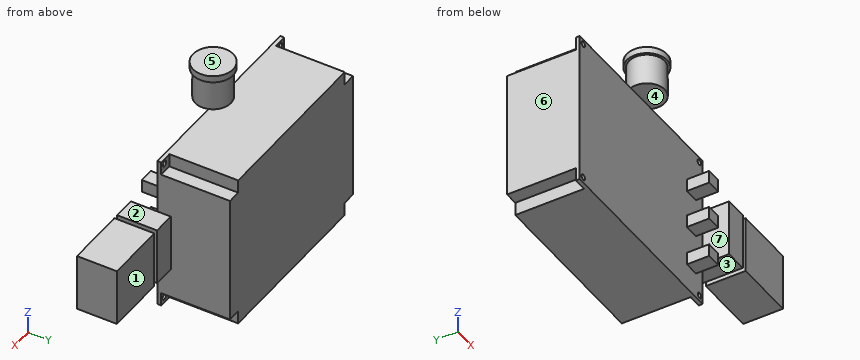
```python
from build123d import *

# Parameters (mm, degrees)
SKETCH2_W               = 90
SKETCH2_H               = 70
BOSS_EXTRUDE1_DEPTH     = 32.6
SKETCH4_R               = 8
BOSS_EXTRUDE2_DEPTH     = 14
SKETCH6_W               = 6.6
SKETCH6_H               = 5.7
BOSS_EXTRUDE3_DEPTH     = 10
SKETCH10_W              = 6.6
SKETCH10_H              = 5.7
BOSS_EXTRUDE4_DEPTH     = 10
SKETCH7_W               = 6.6
SKETCH7_H               = 5.7
BOSS_EXTRUDE5_DEPTH     = 10
CUT_EXTRUDE1_DEPTH      = 122.916565322
CUT_EXTRUDE1_DEPTH_BACK = 122.916565322
SKETCH11_R              = 1.25
CUT_EXTRUDE2_DEPTH      = 122.916565322
CUT_EXTRUDE2_DEPTH_BACK = 122.916565322
SKETCH15_R              = 1.25
CUT_EXTRUDE3_DEPTH      = 122.916565322
CUT_EXTRUDE3_DEPTH_BACK = 122.916565322
SKETCH14_R              = 1.25
CUT_EXTRUDE4_DEPTH      = 122.916565322
CUT_EXTRUDE4_DEPTH_BACK = 122.916565322
SKETCH12_R              = 1.25
SKETCH16_W              = 6
SKETCH16_H              = 6
CUT_EXTRUDE5_DEPTH      = 30.9
SKETCH19_W              = 6
SKETCH19_H              = 6
CUT_EXTRUDE6_DEPTH      = 30.9
SKETCH18_W              = 6
SKETCH18_H              = 6
CUT_EXTRUDE7_DEPTH      = 30.9
SKETCH17_W              = 6
SKETCH17_H              = 6
CUT_EXTRUDE8_DEPTH      = 30.9
SKETCH20_W              = 25.8
SKETCH20_H              = 17.9
BOSS_EXTRUDE6_DEPTH     = 39.4
SKETCH22_W              = 2.1
SKETCH22_H              = 17.9
CUT_EXTRUDE9_DEPTH      = 2.75
SKETCH24_W              = 2.1
SKETCH24_H              = 25.8
CUT_EXTRUDE10_DEPTH     = 2.75
SKETCH25_W              = 2.1
SKETCH25_H              = 17.9
CUT_EXTRUDE11_DEPTH     = 2.75
SKETCH26_W              = 2.1
SKETCH26_H              = 25.8
CUT_EXTRUDE12_DEPTH     = 2.75
SKETCH27_R              = 9
BOSS_EXTRUDE7_DEPTH     = 3


with BuildPart() as part:
    # Sketch2 → Boss-Extrude1 (new body)
    with BuildSketch(Plane(origin=(0, 0, 0), x_dir=(1, 0, 0), z_dir=(0, 1, 0))):
        with Locations((45, 35)):
            Rectangle(SKETCH2_W, SKETCH2_H)
    extrude(amount=BOSS_EXTRUDE1_DEPTH)

    # Sketch4 → Boss-Extrude2 (add)
    with BuildSketch(Plane.XY):
        with Locations(Location((45, -2.57, 0), (0, 0, 161.261463564))):
            Circle(SKETCH4_R)
    extrude(amount=BOSS_EXTRUDE2_DEPTH)

    # Sketch6 → Boss-Extrude3 (add)
    with BuildSketch(Plane(origin=(0, 0, 0), x_dir=(-1, 0, 0), z_dir=(0, -1, 0))):
        with Locations((-81.82, 55.55)):
            Rectangle(SKETCH6_W, SKETCH6_H)
    extrude(amount=BOSS_EXTRUDE3_DEPTH)

    # Sketch10 → Boss-Extrude4 (add)
    with BuildSketch(Plane.XZ):
        with Locations((81.82, -37.25)):
            Rectangle(SKETCH10_W, SKETCH10_H)
    extrude(amount=BOSS_EXTRUDE4_DEPTH)

    # Sketch7 → Boss-Extrude5 (add)
    with BuildSketch(Plane.XZ):
        with Locations((81.82, -19.65)):
            Rectangle(SKETCH7_W, SKETCH7_H)
    extrude(amount=BOSS_EXTRUDE5_DEPTH)

    # Sketch11 → Cut-Extrude1 (cut, two sides: drawn at the far end of the back side and taken through both)
    with BuildSketch(Plane(origin=(0, 32.6, 0), x_dir=(1, 0, 0), z_dir=(0, 1, 0)).offset(-CUT_EXTRUDE1_DEPTH_BACK)):
        with Locations(Location((87.55, 2.29, 0), (0, 0, 90))):
            Circle(SKETCH11_R)
    extrude(amount=CUT_EXTRUDE1_DEPTH + CUT_EXTRUDE1_DEPTH_BACK, mode=Mode.SUBTRACT)

    # Sketch15 → Cut-Extrude2 (cut, two sides: drawn at the far end of the back side and taken through both)
    with BuildSketch(Plane(origin=(0, 32.6, 0), x_dir=(1, 0, 0), z_dir=(0, 1, 0)).offset(-CUT_EXTRUDE2_DEPTH_BACK)):
        with Locations(Location((2.61, 67.35, 0), (0, 0, 90))):
            Circle(SKETCH15_R)
    extrude(amount=CUT_EXTRUDE2_DEPTH + CUT_EXTRUDE2_DEPTH_BACK, mode=Mode.SUBTRACT)

    # Sketch14 → Cut-Extrude3 (cut, two sides: drawn at the far end of the back side and taken through both)
    with BuildSketch(Plane(origin=(0, 32.6, 0), x_dir=(1, 0, 0), z_dir=(0, 1, 0)).offset(-CUT_EXTRUDE3_DEPTH_BACK)):
        with Locations(Location((2.63, 2.25, 0), (0, 0, 90))):
            Circle(SKETCH14_R)
    extrude(amount=CUT_EXTRUDE3_DEPTH + CUT_EXTRUDE3_DEPTH_BACK, mode=Mode.SUBTRACT)

    # Sketch12 → Cut-Extrude4 (cut, two sides: drawn at the far end of the back side and taken through both)
    with BuildSketch(Plane(origin=(0, 32.6, 0), x_dir=(1, 0, 0), z_dir=(0, 1, 0)).offset(-CUT_EXTRUDE4_DEPTH_BACK)):
        with Locations(Location((87.71, 67.37, 0), (0, 0, 90))):
            Circle(SKETCH12_R)
    extrude(amount=CUT_EXTRUDE4_DEPTH + CUT_EXTRUDE4_DEPTH_BACK, mode=Mode.SUBTRACT)

    # Sketch16 → Cut-Extrude5 (cut)
    with BuildSketch(Plane(origin=(0, 32.6, 0), x_dir=(1, 0, 0), z_dir=(0, 1, 0))):
        with Locations((3, 67)):
            Rectangle(SKETCH16_W, SKETCH16_H)
    extrude(amount=-CUT_EXTRUDE5_DEPTH, mode=Mode.SUBTRACT)

    # Sketch19 → Cut-Extrude6 (cut)
    with BuildSketch(Plane(origin=(0, 32.6, 0), x_dir=(1, 0, 0), z_dir=(0, 1, 0))):
        with Locations((3, 3)):
            Rectangle(SKETCH19_W, SKETCH19_H)
    extrude(amount=-CUT_EXTRUDE6_DEPTH, mode=Mode.SUBTRACT)

    # Sketch18 → Cut-Extrude7 (cut)
    with BuildSketch(Plane(origin=(0, 32.6, 0), x_dir=(1, 0, 0), z_dir=(0, 1, 0))):
        with Locations((87, 3)):
            Rectangle(SKETCH18_W, SKETCH18_H)
    extrude(amount=-CUT_EXTRUDE7_DEPTH, mode=Mode.SUBTRACT)

    # Sketch17 → Cut-Extrude8 (cut)
    with BuildSketch(Plane(origin=(0, 32.6, 0), x_dir=(1, 0, 0), z_dir=(0, 1, 0))):
        with Locations((87, 67)):
            Rectangle(SKETCH17_W, SKETCH17_H)
    extrude(amount=-CUT_EXTRUDE8_DEPTH, mode=Mode.SUBTRACT)

    # Sketch20 → Boss-Extrude6 (add)
    with BuildSketch(Plane(origin=(90, 0, 0), x_dir=(0, 0, -1), z_dir=(1, 0, 0))):
        with Locations((37.6, -2.95)):
            Rectangle(SKETCH20_W, SKETCH20_H)
    extrude(amount=BOSS_EXTRUDE6_DEPTH)

    # Sketch22 → Cut-Extrude9 (cut)
    with BuildSketch(Plane(origin=(0, 0, -50.5), x_dir=(-1, 0, 0), z_dir=(0, 0, -1))):
        with Locations((-101.05, -2.95)):
            Rectangle(SKETCH22_W, SKETCH22_H)
    extrude(amount=-CUT_EXTRUDE9_DEPTH, mode=Mode.SUBTRACT)

    # Sketch24 → Cut-Extrude10 (cut)
    with BuildSketch(Plane(origin=(0, 6, 0), x_dir=(1, 0, 0), z_dir=(0, 1, 0))):
        with Locations((101.05, 37.6)):
            Rectangle(SKETCH24_W, SKETCH24_H)
    extrude(amount=-CUT_EXTRUDE10_DEPTH, mode=Mode.SUBTRACT)

    # Sketch25 → Cut-Extrude11 (cut)
    with BuildSketch(Plane.XY.offset(-24.7)):
        with Locations((101.05, -2.95)):
            Rectangle(SKETCH25_W, SKETCH25_H)
    extrude(amount=-CUT_EXTRUDE11_DEPTH, mode=Mode.SUBTRACT)

    # Sketch26 → Cut-Extrude12 (cut)
    with BuildSketch(Plane(origin=(0, -11.9, 0), x_dir=(-1, 0, 0), z_dir=(0, -1, 0))):
        with Locations((-101.05, 37.6)):
            Rectangle(SKETCH26_W, SKETCH26_H)
    extrude(amount=-CUT_EXTRUDE12_DEPTH, mode=Mode.SUBTRACT)

    # Sketch27 → Boss-Extrude7 (add)
    with BuildSketch(Plane.XY.offset(14)):
        with Locations((45, -2.57)):
            Circle(SKETCH27_R)
    extrude(amount=BOSS_EXTRUDE7_DEPTH)


solid = part.part
```
Check sheet for the modelled part. Datum: model origin and axes. Units: mm. Face numbers are marked on the shaded views. A direction names the side the tool comes from. Coordinates: 2 decimals unless noted, no trailing zeros. Loops run counter-clockwise (first coordinate to the right, second up) from the corner with the lowest first, then second, coordinate; pieces in that order, holes last. Notation, with made-up numbers: M 81.25,-9 L 93.25,-9 A8 ccw 93.25,6 Z; hole C 20,76.5 d7. An arc over 180 degrees is marked long. Answer as a JSON object with one key per item and string values.
1. Access from +Z, -Z, +X, -X, +Y, -Y to the whole of each face (thin tool, end or side, straight path). Record for the marked faces 1, 2, 3 and 4.
Outcome:
{"face 1": "+Z, -Z, +X, +Y", "face 2": "+Z, +X, +Y, -Y", "face 3": "-Z, +X, +Y, -Y", "face 4": "-Z, +X, -X, -Y"}
2. Sectioned sample at C-C on x = 45. Record the cut outline in (y, z), and give its area (3 significant figures).
Outcome:
{"outline": "M -11.57,14 L -10.57,14 L -10.57,0 L 0,0 L 0,-70 L 32.6,-70 L 32.6,0 L 5.43,0 L 5.43,14 L 6.43,14 L 6.43,17 L -11.57,17 Z", "area": "2,560 mm²"}
3. Sectioned sample at A-A on y = -2.57. Count the separate pieces of the cut face and the enclosed holes in it, and give its area (3 significant figures).
Outcome:
{"separate pieces": "5", "enclosed holes": "0", "area": "1,400 mm²"}
4. Sectioned sample at B-B on z = -46. Record the cut outline in (x, y).
Outcome:
{"outline": "M 0,0 L 90,0 L 90,-11.9 L 100,-11.9 L 100,-9.15 L 102.1,-9.15 L 102.1,-11.9 L 129.4,-11.9 L 129.4,6 L 102.1,6 L 102.1,3.25 L 100,3.25 L 100,6 L 90,6 L 90,32.6 L 0,32.6 Z"}
5. Sectioned sample at D-D on y = 27. Record the cut outline in (x, z).
Outcome:
{"outline": "M 0,-64 L 6,-64 L 6,-70 L 84,-70 L 84,-64 L 90,-64 L 90,-6 L 84,-6 L 84,0 L 6,0 L 6,-6 L 0,-6 Z"}
6. Release check for a two-part mould opening along X. For the marked faces 5, 6 and 7 record: pulls with the +X half, pulls with the -X half, needs draft (parallel to the pull), parting line crosses it, or undercut.
Outcome:
{"face 5": "needs draft", "face 6": "pulls with the -X half", "face 7": "undercut"}
7. Depth check by flat-ended pin: P1, Ø1.8, axis at y = 23, z = -67.5, coming from the -X side; P2, Ø4, axis at y = 13.5, z = -45, coming from the +X side; P3, Ø1.5, axis at x = 42.5, z = -5.5, coming from the -Y side; P4, Ø3, axis at y = 20.5, z = -57, coming from the -X side. Enter the tip coordinate at first touch or a pass-through.
Outcome:
{"P1": "x = 6", "P2": "x = 90", "P3": "y = 0", "P4": "x = 0"}
8. Scan lines: L1, parallel to X at y = 0.5, z = -67.37; L2, parallel to X at y = 0.8, z = -2.25; L3, parallel to Y at x = 76, z = -57. Record each from-to range of solid material in increasing order. Write a range as from..to.
Outcome:
{"L1": "0..1.36, 3.86..86.46, 88.96..90", "L2": "0..1.38, 3.88..86.3, 88.8..90", "L3": "0..32.6"}
